from build123d import *

# Parameters (mm, degrees)
MODEL_R                 = 10.5
MODEL_R_2               = 3
SALIENTE_EXTRUIR1_DEPTH = 2
CORTAR_EXTRUIR1_REACH   = 4
CROQUIS2_R              = 1.5
CROQUIS3_R              = 4.000000302
CROQUIS3_R_2            = 3
SALIENTE_EXTRUIR2_DEPTH = 2


with BuildPart() as part:
    # Model → Saliente-Extruir1 (new body)
    with BuildSketch(Plane.XY):
        with Locations((162.8, 159.569296)):
            Circle(MODEL_R)
        with Locations((162.8, 159.569296)):
            Circle(MODEL_R_2, mode=Mode.SUBTRACT)
    extrude(amount=SALIENTE_EXTRUIR1_DEPTH)

    # Croquis2 → Cortar-Extruir1 (cut, up to next)
    with BuildSketch(Plane.XY.offset(2), mode=Mode.PRIVATE) as cortar_extruir1_sk1:
        with Locations((156.57897681, 163.758432659)):
            Circle(CROQUIS2_R)
    cortar_extruir1_tool1 = extrude(cortar_extruir1_sk1.sketch, amount=-CORTAR_EXTRUIR1_REACH, mode=Mode.PRIVATE) & part.part
    add(cortar_extruir1_tool1.solids().sort_by_distance((156.578977, 163.758433, 2))[0], mode=Mode.SUBTRACT)
    # Croquis2 → Cortar-Extruir1 (cut, up to next)
    with BuildSketch(Plane.XY.offset(2), mode=Mode.PRIVATE) as cortar_extruir1_sk2:
        with Locations((169.021023816, 155.380159191)):
            Circle(CROQUIS2_R)
    cortar_extruir1_tool2 = extrude(cortar_extruir1_sk2.sketch, amount=-CORTAR_EXTRUIR1_REACH, mode=Mode.PRIVATE) & part.part
    add(cortar_extruir1_tool2.solids().sort_by_distance((169.021024, 155.380159, 2))[0], mode=Mode.SUBTRACT)

    # Croquis3 → Saliente-Extruir2 (add)
    with BuildSketch(Plane.XY.offset(2)):
        with Locations((162.8, 159.569296)):
            Circle(CROQUIS3_R)
        with Locations((162.8, 159.569296)):
            Circle(CROQUIS3_R_2, mode=Mode.SUBTRACT)
    extrude(amount=SALIENTE_EXTRUIR2_DEPTH)


solid = part.part
Verification items for the finished model (mm, model axes). A direction names the side the tool comes from. Coordinates: 2 decimals unless noted, no trailing zeros. Write each loop counter-clockwise with the first axis right and the second up, starting at its lowest first coordinate (ties: lowest second). Pieces come first, ordered by that corner, then holes. Notation, with made-up numbers: (-0.75, 42.25) -> (46.25, 42.25) arc R14 cw to (46.25, 54.25) -> close; hole circle Ø8 at (48.25, 40). An arc over 180 degrees is marked (long way). One line per item, written item: value. Start each with the question number.
Q1. Cross-section at B-B on y = 160.5. Enter the section's corners in (x, z), and give its area (3 significant figures).
Q2. Cross-section at C-C on z = 3. Enter the section's corners in (x, y).
Q3. Thickness scan on L1, parallel to Z at x = 158.75, y = 161.25; L2, parallel to Y at x = 169.5, z = 0.3; L3, parallel to Y at x = 160.75, z = 3.3. Record the ranges inside material, lowest first. Write a range as from..to.
Q4. Cross-section at A-A on x = 162.8. Enter the section's corners in (y, z), and give its area (3 significant figures).
Q5. Access from +Z, -Z, +X, -X, +Y, -Y to the whole of each face (thin tool, end or side, straight path). Record for faces 4 (the cylindrical face through (156.384, 165.246, 1.014)), 5 (the cylindrical face through (158.804, 159.745, 2.986)).
Q6. Mould release check, pull along Y, two halves, no side actions. Record for faces 1 (the cylindrical face through (161.43, 169.98, 0.99)), 2 (the flat face through (163, 155, 2)), 3 (the cylindrical face through (159.803, 159.701, 1.972)): pulls with the +Y half, pulls with the -Y half, needs draft (parallel to the pull), parting line crosses it, or undercut.
Q7. Go/stop test with a flat-tipped pin: P1, Ø1.5, axis at x = 167, y = 153.5, coming from the +Z side. Record where the tip stops, or that it passes through.
Q8. Cross-section at D-D on x = 168.5. Enter the section's corners in (y, z), and give its area (3 significant figures).
Checked values:
1. outline: (152.34, 0) -> (159.95, 0) -> (159.95, 4) -> (158.91, 4) -> (158.91, 2) -> (152.34, 2) -> close; (165.65, 0) -> (173.26, 0) -> (173.26, 2) -> (166.69, 2) -> (166.69, 4) -> (165.65, 4) -> close
1. area: 34.6 mm²
2. outline: circle Ø8 at (162.8, 159.57); hole circle Ø6 at (162.8, 159.57)
3. L1: z = 0..2
3. L2: y = 151.48..153.96, 156.8..167.65
3. L3: y = 156.13..157.38, 161.76..163
4. outline: (149.07, 0) -> (156.57, 0) -> (156.57, 4) -> (155.57, 4) -> (155.57, 2) -> (149.07, 2) -> close; (162.57, 0) -> (170.07, 0) -> (170.07, 2) -> (163.57, 2) -> (163.57, 4) -> (162.57, 4) -> close
4. area: 34.0 mm²
5. face 4: +Z, -Z
5. face 5: +Z
6. face 1: parting line crosses it
6. face 2: needs draft
6. face 3: undercut
7. P1: stops at z = 2
8. outline: (150.75, 0) -> (153.97, 0) -> (153.97, 2) -> (150.75, 2) -> close; (156.79, 0) -> (168.39, 0) -> (168.39, 2) -> (156.79, 2) -> close
8. area: 29.6 mm²
